The model under review builds one solid part; all positions refer to its coordinate system, in mm. Round coordinates to 2 decimals unless told otherwise and drop trailing zeros. Order: outer loops, then holes, each group sorted by start corner. A loop starts at its lowest first (then second) coordinate and runs counter-clockwise, first axis right, second up. Notation, with made-up numbers: (63, 15.25) - (70, 15.25) arc R18 cw to (70, 23.25) - close; hole circle Ø2 at (31, -23). An arc over 180 degrees is marked (long way). One line per question, with ' | ' between items. Start each with the question number.
Item 1: Add section A-A on x = -9.5. State how many separate pieces and enclosed holes the cut face has, and give its area (3 significant figures).
Item 2: Add section D-D on y = -19. State the section outline as (x, z) points, and give its area (3 significant figures).
Item 3: For L1, parallel to X at y = -5.5, z = 1.6; L2, parallel to Y at x = 27, z = 1.8; L3, parallel to Z at x = 11, y = -27, list the stretches that pass through material, from the lowest coordinate up. Write a range as [from, to].
Item 4: Insertion check: pin 1 Ø1 at (x, y) = (-1.5, -32) entering from +Z; pin 2 Ø0.9 at (y, z) = (-20, 4) entering from +X; pin 3 Ø2.5 at (x, z) = (8, 4.5) entering from +Y. Each pin has a flat end and moves straight along its axis. Give the tip position at first contact, or say it passes through.
Item 5: Add section B-B on y = -4. State the section outline as (x, z) points, and give its area (3 significant figures).
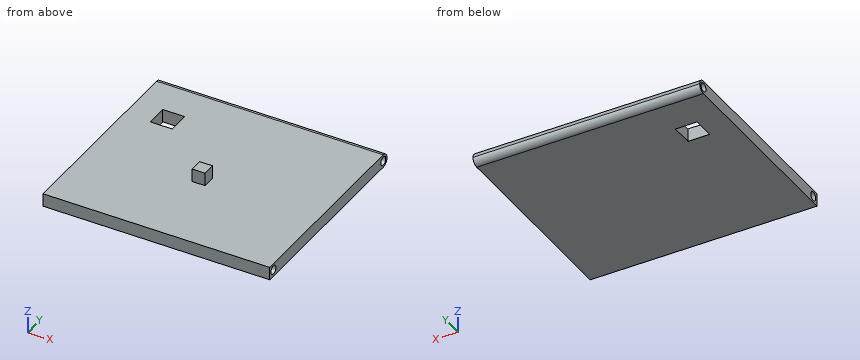
from build123d import *

# Parameters (mm, degrees)
SKETCH_1_W          = 52
SKETCH_1_H          = 47
EXTRUDE_1_DEPTH     = 3
SKETCH_2_R          = 1
CUT_EXTRUDE_1_DEPTH = 92
FILLET_1_R          = 1.5
FILLET_2_R          = 1.5
SKETCH_3_R          = 1
CUT_EXTRUDE_2_DEPTH = 92
SKETCH_4_W          = 3
SKETCH_4_H          = 3
EXTRUDE_2_DEPTH     = 3
SKETCH_5_W          = 5
SKETCH_5_H          = 5
CUT_EXTRUDE_3_DEPTH = 6


with BuildPart() as part:
    # 草图1 → 凸台-拉伸1 (new body)
    with BuildSketch(Plane.XY):
        with Locations((9.526717557, -16.255725191)):
            Rectangle(SKETCH_1_W, SKETCH_1_H)
    extrude(amount=EXTRUDE_1_DEPTH)

    # 草图2 → 切除-拉伸1 (cut)
    with BuildSketch(Plane(origin=(35.526717557, 0, 0), x_dir=(0, 0, -1), z_dir=(1, 0, 0))):
        with Locations(Location((-1.5, 5.744274809, 0), (0, 0, 90))):
            Circle(SKETCH_2_R)
    extrude(amount=-CUT_EXTRUDE_1_DEPTH, mode=Mode.SUBTRACT)

    # 圆角1
    fillet_1_edges = [part.edges().sort_by_distance(p)[0] for p in [
        (9.526717557, 7.244274809, 0),
    ]]
    fillet(fillet_1_edges, radius=FILLET_1_R)

    # 圆角2
    fillet_2_edges = [part.edges().sort_by_distance(p)[0] for p in [
        (9.526717557, 7.244274809, 3),
    ]]
    fillet(fillet_2_edges, radius=FILLET_2_R - 0.0001)  # a hair under: the kernel refuses the full size

    # 草图3 → 切除-拉伸2 (cut)
    with BuildSketch(Plane(origin=(35.526717557, 0, 0), x_dir=(0, 0, -1), z_dir=(1, 0, 0))):
        with Locations(Location((-1.5, -38.255725191, 0), (0, 0, 90))):
            Circle(SKETCH_3_R)
    extrude(amount=-CUT_EXTRUDE_2_DEPTH, mode=Mode.SUBTRACT)

    # 草图4 → 凸台-拉伸2 (add)
    with BuildSketch(Plane.XY.offset(3)):
        with Locations((8.626717557, -19.755725191)):
            Rectangle(SKETCH_4_W, SKETCH_4_H)
    extrude(amount=EXTRUDE_2_DEPTH)

    # 草图5 → 切除-拉伸3 (cut)
    with BuildSketch(Plane(origin=(0, 0, 0), x_dir=(-1, 0, 0), z_dir=(0, 0, -1))):
        with Locations((7.973282443, -4.755725191)):
            Rectangle(SKETCH_5_W, SKETCH_5_H)
    extrude(amount=-CUT_EXTRUDE_3_DEPTH, mode=Mode.SUBTRACT)


solid = part.part
Determined:
1) separate pieces: 2 | enclosed holes: 2 | area: 119 mm2
2) outline: (-16.47, 0) - (35.53, 0) - (35.53, 3) - (10.13, 3) - (10.13, 6) - (7.13, 6) - (7.13, 3) - (-16.47, 3) - close | area: 165 mm2
3) L1: [-16.47, -10.47], [-5.47, 35.53] | L2: [-39.76, -39.21], [-37.3, 4.79], [6.7, 7.21] | L3: [0, 3]
4) pin 1: z = 3 | pin 2: x = 10.13 | pin 3: y = -18.26
5) outline: (-16.47, 0) - (-10.47, 0) - (-10.47, 3) - (-16.47, 3) - close; (-5.47, 0) - (35.53, 0) - (35.53, 3) - (-5.47, 3) - close | area: 141 mm2
